from build123d import *

# Parameters (mm, degrees)
SKETCH1_R           = 1.5
BOSS_EXTRUDE1_DEPTH = 165


with BuildPart() as part:
    # Sketch1 → Boss-Extrude1 (new body)
    with BuildSketch(Plane(origin=(0, 0, 0), x_dir=(1, 0, 0), z_dir=(0, 1, 0))):
        with BuildLine():
            Line((-30.194572404, -4.825127674), (-30.194572404, 3.170664552))
            Line((-30.194572404, 3.170664552), (-19.637232632, 3.170664552))
            Line((-19.637232632, 3.170664552), (-17.713971419, 3.170664552))
            ThreePointArc((-17.713971419, 3.170664552), (-15.592651075, 2.291984895), (-14.713971419, 0.170664552))
            Line((-14.713971419, 0.170664552), (-14.713971419, -1.825127674))
            ThreePointArc((-14.713971419, -1.825127674), (-15.592651075, -3.946448018), (-17.713971419, -4.825127674))
            Line((-17.713971419, -4.825127674), (-30.194572404, -4.825127674))
        make_face()
        with Locations((-20.713971419, -0.825127674)):
            Circle(SKETCH1_R, mode=Mode.SUBTRACT)
        with Locations((-26.713971419, -0.825127674)):
            Circle(SKETCH1_R, mode=Mode.SUBTRACT)
    extrude(amount=BOSS_EXTRUDE1_DEPTH)


solid = part.part
The model under review builds one solid part; all positions refer to its coordinate system, in mm. Give positions to 0.01 mm unless a question says otherwise; leave off trailing zeros. Loops run counter-clockwise (first coordinate to the right, second up) from the corner with the lowest first, then second, coordinate; pieces in that order, holes last. Notation, with made-up numbers: (-8, 42.5) -> (24, 42.5) arc R15 cw to (24, 65.5) -> close; hole circle Ø2 at (37, 59.25). An arc over 180 degrees is marked (long way). Put each result on its own line as item: value. Start each with the question number.
1. Mouldability with a two-part tool opening along Z and no side actions: class faces 1 (the face through (-19.283, 81.345, 0.375)), 2 (the face through (-15.569, 81.345, 3.923)), 3 (the face through (-22.3, 165, -0.1)), 4 (the face through (-15.6, 81.3, -2.3)) as released by +Z, released by -Z, zero draft, split by the parting line, or undercut.
2. We need section A-A on y = 68. State the section outline as (x, z) points, then the cut area to 3 significant figures.
3. Clearance check with a flat-ended pin moving along its axis: P1, Ø2, axis at y = 82.5, z = 3.5, coming from the +X side. State where the tip first meets the part, or that it passes through.
4. Wall thickness on probe 1 along X at (y, z) = (9.5, 1); probe 2 along X at (y, z) = (59, -0.25); probe 3 along Z at (x, y) = (-21, 17.5): over which ranges is each line inside the solid? List them lowest first.
Determined:
1. face 1: undercut
1. face 2: released by +Z
1. face 3: zero draft
1. face 4: released by -Z
2. outline: (-30.19, -3.17) -> (-17.71, -3.17) arc R3 ccw to (-14.71, -0.17) -> (-14.71, 1.83) arc R3 ccw to (-17.71, 4.83) -> (-30.19, 4.83) -> close; hole circle Ø3 at (-26.71, 0.83); hole circle Ø3 at (-20.71, 0.83)
2. area: 106 mm^2
3. P1: x = -14.79
4. probe 1: -30.19 to -28.2, -25.22 to -22.2, -19.22 to -14.71
4. probe 2: -30.19 to -27.76, -25.67 to -21.76, -19.67 to -14.72
4. probe 3: -3.17 to -0.65, 2.3 to 4.83
